```python
from build123d import *

# Parameters (mm, degrees)
F0_R      = 18.03
F1_DEPTH  = 20.701
F3_R      = 20.545
F4_DEPTH  = 17.272
F6_R      = 17.525
F7_DEPTH  = 27.35
F9_R      = 23.115
F10_DEPTH = 17.27
F12_R     = 21.5
F13_DEPTH = 40


with BuildPart() as f1:
    # F0 (on Front) → F1 (new body)
    with BuildSketch(Plane.XZ):
        Circle(F0_R)
    extrude(amount=-F1_DEPTH)

    # F3 (on offset) → F4 (join)
    with BuildSketch(Plane(origin=(0, 20.701, 0), x_dir=(1, 0, 0), z_dir=(0, 1, 0))):
        Circle(F3_R)
    extrude(amount=F4_DEPTH)

    # F6 (on offset) → F7 (join)
    with BuildSketch(Plane(origin=(0, 37.973, 0), x_dir=(1, 0, 0), z_dir=(0, 1, 0))):
        Circle(F6_R)
    extrude(amount=F7_DEPTH)

    # F9 (on offset) → F10 (join)
    with BuildSketch(Plane(origin=(0, 65.323, 0), x_dir=(1, 0, 0), z_dir=(0, 1, 0))):
        Circle(F9_R)
    extrude(amount=F10_DEPTH)

    # F12 (on offset) → F13 (join)
    with BuildSketch(Plane(origin=(0, 82.593, 0), x_dir=(1, 0, 0), z_dir=(0, 1, 0))):
        Circle(F12_R)
    extrude(amount=F13_DEPTH)


solid = f1.part
```
Work out the finished part from the listing and answer in its coordinate system (mm). A direction names the side the tool comes from. Round coordinates to 2 decimals unless told otherwise and drop trailing zeros. Loops run counter-clockwise (first coordinate to the right, second up) from the corner with the lowest first, then second, coordinate; pieces in that order, holes last.
(1) The part is cut by section B-B, the plane z = 0. Give the vertices of the cut face in (x, y) (3 decimals).
Computed values:
outline: (-23.115, 65.323) - (-17.525, 65.323) - (-17.525, 37.973) - (-20.545, 37.973) - (-20.545, 20.701) - (-18.03, 20.701) - (-18.03, 0) - (18.03, 0) - (18.03, 20.701) - (20.545, 20.701) - (20.545, 37.973) - (17.525, 37.973) - (17.525, 65.323) - (23.115, 65.323) - (23.115, 82.593) - (21.5, 82.593) - (21.5, 122.593) - (-21.5, 122.593) - (-21.5, 82.593) - (-23.115, 82.593) - close
(2) The part is cut by section D-D, the plane y = 76.5. Give the vertices of the cut face in (x, z) (3 decimals), and give its area (3 significant figures).
Computed values:
outline: circle Ø46.23 at (0, 0)
area: 1,680 mm2
(3) Each of these flat-tipped pins is pushed along its axis until it touches: P1, Ø8, axis at x = -3.5, y = 54.5, coming from the -Z side (3 decimals); P2, Ø10, axis at x = 4.5, y = 14.5, coming from the +Z side; P3, Ø10, axis at x = 14.5, y = 46, coming from the +Z side. Where does it stop, or does it pass through?
Computed values:
P1: stops at z = -17.525
P2: stops at z = 18.03
P3: stops at z = 14.73
(4) For faces 1 (the cylindrical face through (-14.31, 10.21, -10.97)), 2 (the cylindrical face through (-2.281, 51.457, -17.376)), 3 (the cylindrical face through (-2.799, 102.313, -21.317)), determine the directions among +Z, -Z, +X, -X, +Y, -Y from which every point of the face is accessible in a straight line to the end or side of a thin tool.
Computed values:
face 1: -Y
face 2: none
face 3: +Y
(5) The mould has two halves that part along Y. Classify faces 4 (the flat face through (17, 82.593, 14)), 5 (the flat face through (15.1, 37.973, -9.2)), 6 (the flat face through (0, 0, 0)), 7 (the cylindrical face through (-5.011, 73.837, 22.565)): pulls with the +Y half, pulls with the -Y half, needs draft (parallel to the pull), parting line crosses it, or undercut.
Computed values:
face 4: pulls with the +Y half
face 5: undercut
face 6: pulls with the -Y half
face 7: needs draft
(6) Find the intervals of material crossed by L1, parallel to Y at x = 5, z = 18; L2, parallel to Y at x = 17.5, z = -13; L3, parallel to Z at x = -16.5, y = 19, in increasing order.
Computed values:
L1: y = 20.7 to 37.97, 65.32 to 122.59
L2: y = 65.32 to 82.59
L3: z = -7.27 to 7.27
(7) The part is cut by section A-A, the plane x = 0. Give the vertices of the cut face in (y, z) (3 decimals).
Computed values:
outline: (0, -18.03) - (20.701, -18.03) - (20.701, -20.545) - (37.973, -20.545) - (37.973, -17.525) - (65.323, -17.525) - (65.323, -23.115) - (82.593, -23.115) - (82.593, -21.5) - (122.593, -21.5) - (122.593, 21.5) - (82.593, 21.5) - (82.593, 23.115) - (65.323, 23.115) - (65.323, 17.525) - (37.973, 17.525) - (37.973, 20.545) - (20.701, 20.545) - (20.701, 18.03) - (0, 18.03) - close
(8) The part is cut by section C-C, the plane y = 100. Give the vertices of the cut face in (x, z), and give its area (3 significant figures).
Computed values:
outline: circle Ø43 at (0, 0)
area: 1,450 mm2
